Here's how the part is built. I have some questions about the finished solid (model axes, mm). Coordinates: 2 decimals unless noted, no trailing zeros. Write each loop counter-clockwise with the first axis right and the second up, starting at its lowest first coordinate (ties: lowest second). Pieces come first, ordered by that corner, then holes.
Item 1: I'm going to push a flat-ended pin straight in: pin 1 Ø3 at (x, y) = (187.25, 40.5) entering from -Z. Where does the tip first touch, or does it pass through?
Item 2: If we section it at C-C (x = 12.75): Please give me the cut outline in (y, z), then the cut area to 3 significant figures.
Item 3: If I drill on line 1 (Y direction, x = 28.5, z = 1.05); line 2 (Y direction, x = 187.25, z = 0.6); line 3 (X direction, y = 4, z = 2.95), over which ranges is the centre line in solid material (lowest first)?
Item 4: If we section it at B-B (z = 2.5): Count the separate pieces of the cut face and the enclosed holes in it, then the cut area to 4 significant figures.
Item 5: If we section it at A-A (x = 48.5): Please give me the cut outline in (y, z), then the cut area to 3 significant figures.
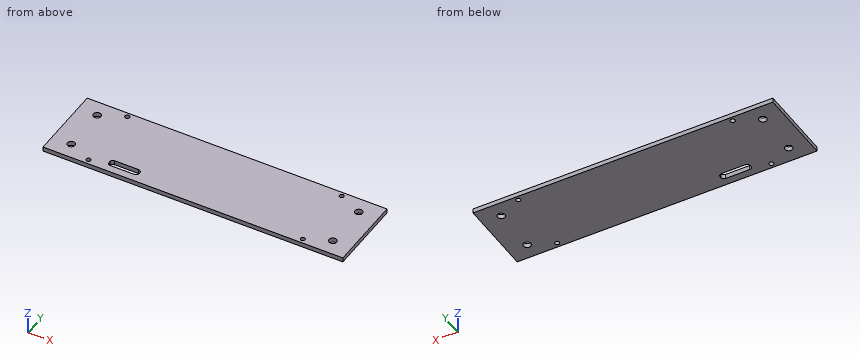
from build123d import *

# Parameters (mm, degrees)
SKETCH1_W           = 200
SKETCH1_H           = 51
BOSS_EXTRUDE1_DEPTH = 3
SKETCH2_R           = 1.5
SKETCH2_R_2         = 2.5
CUT_EXTRUDE1_DEPTH  = 3
SKETCH3_W           = 20
SKETCH3_H           = 5
CUT_EXTRUDE2_DEPTH  = 3
FILLET1_R           = 2


with BuildPart() as part:
    # Sketch1 → Boss-Extrude1 (new body)
    with BuildSketch(Plane.XY):
        with Locations((100, 25.5)):
            Rectangle(SKETCH1_W, SKETCH1_H)
    extrude(amount=BOSS_EXTRUDE1_DEPTH)

    # Sketch2 → Cut-Extrude1 (cut)
    with BuildSketch(Plane.XY.offset(3)):
        with Locations((28.5, 48)):
            Circle(SKETCH2_R)
        with Locations((28.5, 3.25)):
            Circle(SKETCH2_R)
        with Locations((12.75, 40.5)):
            Circle(SKETCH2_R_2)
        with Locations((12.75, 10.5)):
            Circle(SKETCH2_R_2)
        with Locations((187.25, 40.5)):
            Circle(SKETCH2_R_2)
        with Locations((187.25, 10.5)):
            Circle(SKETCH2_R_2)
        with Locations((171.5, 3.25)):
            Circle(SKETCH2_R)
        with Locations((171.5, 48)):
            Circle(SKETCH2_R)
    extrude(amount=-CUT_EXTRUDE1_DEPTH, mode=Mode.SUBTRACT)

    # Sketch3 → Cut-Extrude2 (cut)
    with BuildSketch(Plane.XY.offset(3)):
        with Locations((50, 7.5)):
            Rectangle(SKETCH3_W, SKETCH3_H)
    extrude(amount=-CUT_EXTRUDE2_DEPTH, mode=Mode.SUBTRACT)

    # Fillet1
    fillet1_edges = [part.edges().sort_by_distance(p)[0] for p in [
        (40, 5, 1.5),
        (40, 10, 1.5),
        (60, 10, 1.5),
        (60, 5, 1.5),
    ]]
    fillet(fillet1_edges, radius=FILLET1_R)


solid = part.part
Answer list:
1. pin 1: passes through
2. outline: (0, 0) - (8, 0) - (8, 3) - (0, 3) - close; (13, 0) - (38, 0) - (38, 3) - (13, 3) - close; (43, 0) - (51, 0) - (51, 3) - (43, 3) - close
2. area: 123 mm2
3. line 1: y = 0 to 1.75, 4.75 to 46.5, 49.5 to 51
3. line 2: y = 0 to 8, 13 to 38, 43 to 51
3. line 3: x = 0 to 27.2, 29.8 to 170.2, 172.8 to 200
4. separate pieces: 1
4. enclosed holes: 9
4. area: 10,000 mm2
5. outline: (0, 0) - (5, 0) - (5, 3) - (0, 3) - close; (10, 0) - (51, 0) - (51, 3) - (10, 3) - close
5. area: 138 mm2
